The listing builds one solid part. Answer for the finished solid, in the listing's coordinates (mm). Face numbers are marked on the shaded views. A direction names the side the tool comes from. Coordinates: 2 decimals unless noted, no trailing zeros. Order: outer loops, then holes, each group sorted by start corner. A loop starts at its lowest first (then second) coordinate and runs counter-clockwise, first axis right, second up. Notation, with made-up numbers: (83, 50) -> (126, 50) arc R16 ccw to (126, 55) -> close; hole circle Ø3 at (-38.75, 81). An arc over 180 degrees is marked (long way). Return JSON: item names as keys, results as strings.
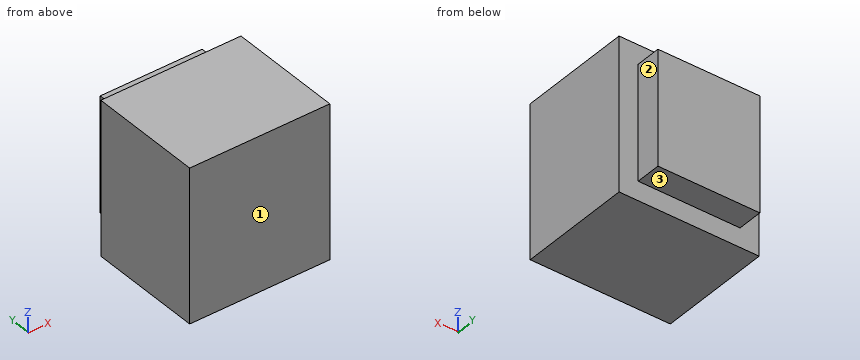
from build123d import *

# Parameters (mm, degrees)
SKETCH_1_W      = 11
SKETCH_1_H      = 12
EXTRUDE_1_DEPTH = 9
SKETCH_2_W      = 8
SKETCH_2_H      = 9
EXTRUDE_2_DEPTH = 2


with BuildPart() as part:
    # Эскиз1 → Бобышка-Вытянуть1 (new body)
    with BuildSketch(Plane(origin=(0, 0, 0), x_dir=(1, 0, 0), z_dir=(0, 1, 0))):
        Rectangle(SKETCH_1_W, SKETCH_1_H)
    extrude(amount=EXTRUDE_1_DEPTH)

    # Эскиз2 → Бобышка-Вытянуть2 (add)
    with BuildSketch(Plane(origin=(0, 9, 0), x_dir=(1, 0, 0), z_dir=(0, 1, 0))):
        Rectangle(SKETCH_2_W, SKETCH_2_H)
    extrude(amount=EXTRUDE_2_DEPTH)


solid = part.part
1. The part is cut by section A-A on z = 0.25. Give the vertices of the cut face in (x, y), and give its area (3 significant figures).
Answer block:
{"outline": "(-5.5, 0) -> (5.5, 0) -> (5.5, 9) -> (4, 9) -> (4, 11) -> (-4, 11) -> (-4, 9) -> (-5.5, 9) -> close", "area": "115 mm2"}
2. For the marked faces 1, 2 and 3, determine the directions among +Z, -Z, +X, -X, +Y, -Y from which every point of the face is accessible in a straight line to the end or side of a thin tool.
Answer block:
{"face 1": "+Z, -Z, +X, -X, -Y", "face 2": "+Z, -Z, +X, +Y", "face 3": "-Z, +X, -X, +Y"}
3. Consider line 1 (X direction, y = 9.75, z = 2.75); line 2 (Z direction, x = -3.5, y = 10.5); line 3 (Y direction, x = -4.5, z = -0.25). Determine where each line is inside the solid, lowest interval first. Write a range as from..to.
Answer block:
{"line 1": "x = -4..4", "line 2": "z = -4.5..4.5", "line 3": "y = 0..9"}
4. The part is cut by section B-B on x = 3.5. Give the vertices of the cut face in (y, z), and give its area (3 significant figures).
Answer block:
{"outline": "(0, -6) -> (9, -6) -> (9, -4.5) -> (11, -4.5) -> (11, 4.5) -> (9, 4.5) -> (9, 6) -> (0, 6) -> close", "area": "126 mm2"}
